```python
from build123d import *

# Parameters (mm, degrees)
SKETCH1_R           = 25.4
BOSS_EXTRUDE1_DEPTH = 25.4
CUT_EXTRUDE1_DEPTH  = 19.05
SKETCH3_R           = 2.8
CUT_EXTRUDE2_DEPTH  = 44.994090512


with BuildPart() as part:
    # Sketch1 → Boss-Extrude1 (new body)
    with BuildSketch(Plane.XY):
        Circle(SKETCH1_R)
    extrude(amount=BOSS_EXTRUDE1_DEPTH)

    # Sketch2 → Cut-Extrude1 (cut)
    with BuildSketch(Plane.XY.offset(25.4)):
        with BuildLine():
            Line((-21.945834457, 13.97), (21.945834457, 13.97))
            ThreePointArc((21.945834457, 13.97), (26.015006247, 0), (21.945834457, -13.97))
            Line((21.945834457, -13.97), (-21.945834457, -13.97))
            ThreePointArc((-21.945834457, -13.97), (-26.015006247, 0), (-21.945834457, 13.97))
        make_face()
    extrude(amount=-CUT_EXTRUDE1_DEPTH, mode=Mode.SUBTRACT)

    # Sketch3 → Cut-Extrude2 (cut, through all)
    with BuildSketch(Plane.XY.offset(25.4)):
        with Locations((0, 17.5)):
            Circle(SKETCH3_R)
        with Locations((0, -17.5)):
            Circle(SKETCH3_R)
    extrude(amount=-CUT_EXTRUDE2_DEPTH, mode=Mode.SUBTRACT)


solid = part.part
```
Verification items for the finished model (mm, model axes). A direction names the side the tool comes from. Round coordinates to 2 decimals unless told otherwise and drop trailing zeros. Write each loop counter-clockwise with the first axis right and the second up, starting at its lowest first coordinate (ties: lowest second). Pieces come first, ordered by that corner, then holes. Notation, with made-up numbers: (-14, 80) -> (39, 80) arc R29 cw to (39, 111) -> close; hole circle Ø10 at (59, -35.5). An arc over 180 degrees is marked (long way). Write each question's results on one line, items separated by ' | '.
Q1. Go/stop test with flat-tipped pins: pin 1 Ø5.5 at (x, z) = (-4.5, 20) entering from +Y; pin 2 Ø22.5 at (x, y) = (-9.5, -2) entering from +Z; pin 3 Ø3 at (x, z) = (-11.5, 11.5) entering from +Y; pin 4 Ø6 at (y, z) = (-6, 10) entering from -X. Record where each tip stops, or that it passes through.
Derived:
pin 1: stops at y = 25.34 | pin 2: stops at z = 6.35 | pin 3: stops at y = 23.35 | pin 4: passes through
Q2. Draft check along X on faces 1 (the face through (-0.607, -20.233, 12.878)), 2 (the face through (0, 0, 6.35)), 3 (the face through (-20.157, -15.456, 12.522)). Enter one of: released by +X, released by -X, zero draft, split by the parting line, or undercut.
Derived:
face 1: undercut | face 2: zero draft | face 3: split by the parting line
Q3. Sectioned sample at A-A, the plane x = 0. Record the boundary of the cut face in (y, z), and give its area (3 significant figures).
Derived:
outline: (-25.4, 0) -> (-20.3, 0) -> (-20.3, 25.4) -> (-25.4, 25.4) -> close; (-14.7, 0) -> (14.7, 0) -> (14.7, 25.4) -> (13.97, 25.4) -> (13.97, 6.35) -> (-13.97, 6.35) -> (-13.97, 25.4) -> (-14.7, 25.4) -> close; (20.3, 0) -> (25.4, 0) -> (25.4, 25.4) -> (20.3, 25.4) -> close | area: 474 mm²
Q4. Sectioned sample at D-D, the plane z = 2.5. Record the boundary of the cut face in (x, y).
Derived:
outline: circle Ø50.8 at (0, 0); hole circle Ø5.6 at (0, -17.5); hole circle Ø5.6 at (0, 17.5)
Q5. Thickness scan on probe 1 along Y at (x, z) = (0, 8); probe 2 along Z at (x, y) = (-19, 11); probe 3 along Y at (x, z) = (9, 9.5). Record the ranges inside material, lowest first.
Derived:
probe 1: y = -25.4 to -20.3, -14.7 to -13.97, 13.97 to 14.7, 20.3 to 25.4 | probe 2: z = 0 to 6.35 | probe 3: y = -23.75 to -13.97, 13.97 to 23.75
Q6. Access from +Z, -Z, +X, -X, +Y, -Y to the whole of each face (thin tool, end or side, straight path). Record for faces 4 (the face through (0, 0, 0)), 5 (the face through (0, 13.97, 16)).
Derived:
face 4: -Z, +X, -X, +Y, -Y | face 5: +Z, +X, -X
Q7. Sectioned sample at B-B, the plane z = 11.5. Record the boundary of the cut face in (x, y), and give its area (3 significant figures).
Derived:
outline: (-21.21, -13.97) arc R25.4 ccw to (21.21, -13.97) -> close; (-21.21, 13.97) -> (21.21, 13.97) arc R25.4 ccw to start; hole circle Ø5.6 at (0, -17.5); hole circle Ø5.6 at (0, 17.5) | area: 633 mm²
Q8. Sectioned sample at C-C, the plane y = -17.5. Record the boundary of the cut face in (x, z).
Derived:
outline: (-18.41, 0) -> (-2.8, 0) -> (-2.8, 25.4) -> (-18.41, 25.4) -> close; (2.8, 0) -> (18.41, 0) -> (18.41, 25.4) -> (2.8, 25.4) -> close
